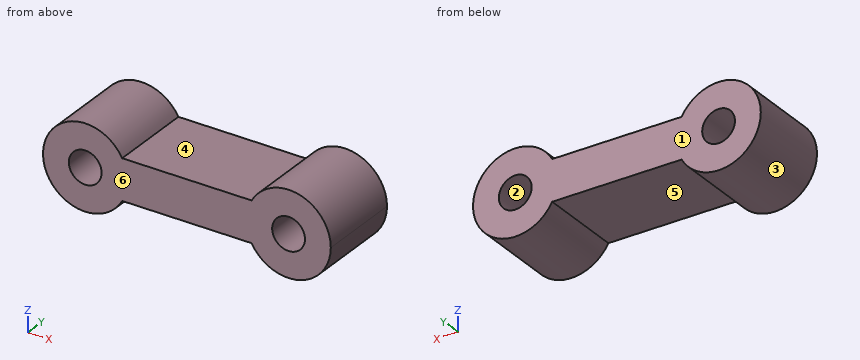
from build123d import *

# Parameters (mm, degrees)
F0_R     = 9.855084
F1_DEPTH = 50.8


with BuildPart() as f1:
    # F0 (on Front) → F1 (new body)
    with BuildSketch(Plane.XZ):
        with BuildLine():
            ThreePointArc((-22.239753, -12.270021), (6.33523, -24.597253), (25.4, 0))
            ThreePointArc((25.4, 0), (6.33523, 24.597253), (-22.239753, 12.270021))
            ThreePointArc((-22.239753, 12.270021), (-25.4, 0), (-22.239753, -12.270021))
        make_face()
        Circle(F0_R, mode=Mode.SUBTRACT)
        with BuildLine():
            ThreePointArc((-96.932443, 0), (-97.73519, 6.33523), (-100.09269, 12.270021))
            ThreePointArc((-100.09269, 12.270021), (-147.732443, 0), (-100.09269, -12.270021))
            ThreePointArc((-100.09269, -12.270021), (-97.73519, -6.33523), (-96.932443, 0))
        make_face()
        with Locations((-122.332443, 0)):
            Circle(F0_R, mode=Mode.SUBTRACT)
        with BuildLine():
            ThreePointArc((-22.239753, -12.270021), (-25.4, 0), (-22.239753, 12.270021))
            Line((-22.239753, 12.270021), (-100.09269, 12.270021))
            ThreePointArc((-100.09269, 12.270021), (-97.73519, 6.33523), (-96.932443, 0))
            ThreePointArc((-96.932443, 0), (-97.73519, -6.33523), (-100.09269, -12.270021))
            Line((-100.09269, -12.270021), (-22.239753, -12.270021))
        make_face()
    extrude(amount=F1_DEPTH)


solid = f1.part
Design review of the part built by this model. Coordinates are the model's own, in mm. Face numbers are marked on the shaded views. A direction names the side the tool comes from. Coordinates: 2 decimals unless noted, no trailing zeros. Loops run counter-clockwise (first coordinate to the right, second up) from the corner with the lowest first, then second, coordinate; pieces in that order, holes last. Notation, with made-up numbers: M 37,71 L 55,71 A5 ccw 55,80 Z; hole C -34,32.25 d8. An arc over 180 degrees is marked long. Answer as CSV lines item,"result".
Item 1: For probe 1 along X at (y, z) = (-6.5, 0.5); probe 2 along X at (y, z) = (-48.5, 4); probe 3 along Z at (x, y) = (-85.5, -37), list the stretches that pass through material, from the lowest coordinate up.
Answer list:
probe 1,"-147.73 to -132.17, -112.49 to -9.84, 9.84 to 25.4"
probe 2,"-147.42 to -131.34, -113.33 to -9.01, 9.01 to 25.08"
probe 3,"-12.27 to 12.27"
Item 2: Add section C-C on y = -9. State the section outline as (x, z) points.
Answer list:
outline,"M -100.09,-12.27 L -22.24,-12.27 A25.4 ccw long -22.24,12.27 L -100.09,12.27 A25.4 ccw long Z; hole C -122.33,0 d19.71; hole C 0,0 d19.71"
Item 3: The part is to be moulded in two halves that separate along Z. For the marked faces 1, 2 and 3, say which applies: pulls with the +Z half, pulls with the -Z half, needs draft (parallel to the pull), parting line crosses it, or undercut.
Answer list:
face 1,"needs draft"
face 2,"undercut"
face 3,"parting line crosses it"
Item 4: Machinability: for the marked faces 4, 5 and 6, which of the approach directions +Z, -Z, +X, -X, +Y, -Y give a long, thin tool a straight path to every point of the face, cutting with its end or side? Answer none if there is none.
Answer list:
face 4,"+Z, +Y, -Y"
face 5,"-Z, +Y, -Y"
face 6,"+Z, -Z, +X, -X, -Y"
Item 5: Add section D-D on z = 14.5. State the section outline as (x, y) points.
Answer list:
outline,"M -143.19,-50.8 L -101.48,-50.8 L -101.48,0 L -143.19,0 Z; M -20.85,-50.8 L 20.85,-50.8 L 20.85,0 L -20.85,0 Z"
Item 6: Add section A-A on x = 0. State the section outline as (y, z) points.
Answer list:
outline,"M -50.8,-25.4 L 0,-25.4 L 0,-9.86 L -50.8,-9.86 Z; M -50.8,9.86 L 0,9.86 L 0,25.4 L -50.8,25.4 Z"
Item 7: Add section B-B on z = -1.5. State the section outline as (x, y) points, plus the area to 3 significant figures.
Answer list:
outline,"M -147.69,-50.8 L -132.07,-50.8 L -132.07,0 L -147.69,0 Z; M -112.59,-50.8 L -9.74,-50.8 L -9.74,0 L -112.59,0 Z; M 9.74,-50.8 L 25.36,-50.8 L 25.36,0 L 9.74,0 Z"
area,"6,810 mm²"
Item 8: For P1, Ø8, axis at y = -37.5, z = 15.5, coming from the -X side; P2, Ø12, axis at x = -122.33, z = 0, coming from the +Y side; P3, Ø5, axis at y = -39.5, z = 3, coming from the +X side; P4, Ø8, axis at x = -47, y = -6, coming from the +Z side, all flat-tipped, find the tip position at first contact; note any pin that passes through.
Answer list:
P1,"x = -144.98"
P2,"through"
P3,"x = 25.4"
P4,"z = 12.27"
